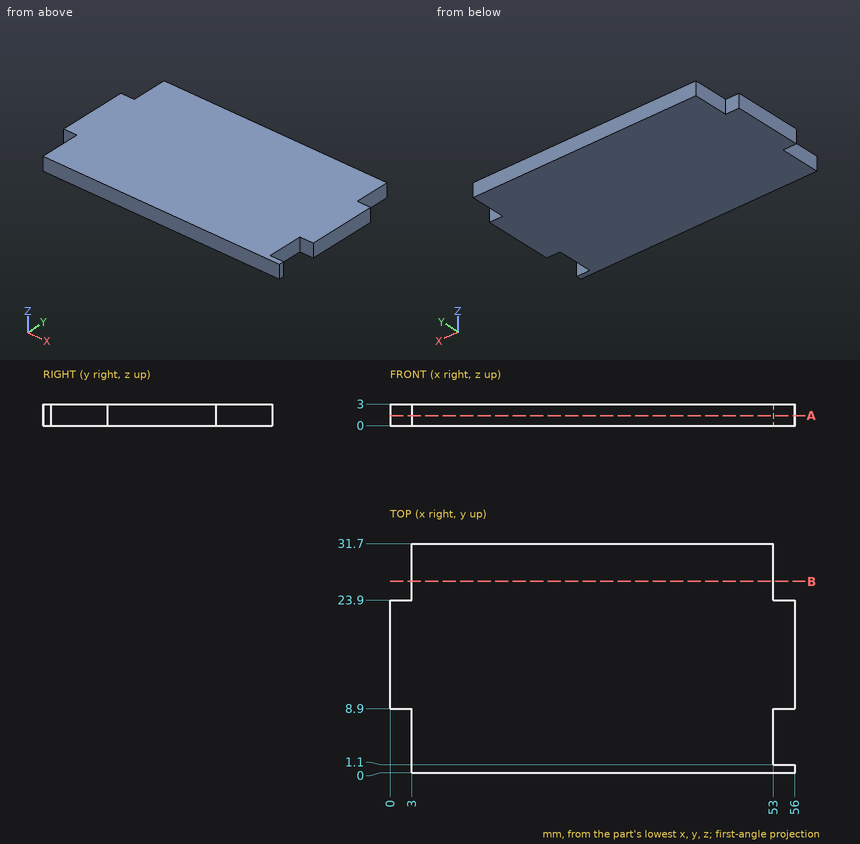
Geometry: see drawing. Coordinates: mm, zero at the bounding-box minimum. Give positions to 0.01 mm unless a question says otherwise; leave off trailing zeros. Write each loop counter-clockwise with the first axis right and the second up, starting at its lowest first coordinate (ties: lowest second). Pieces come first, ordered by that corner, then holes. Notation, with made-up numbers: (43.5, -0.75) -> (75.5, -0.75) arc R31 cw to (75.5, 24.25) -> close; hole circle Ø9 at (46, 4). An arc over 180 degrees is marked (long way). Use one line per item in the form item = value. Start each with the question number.
1) Pin query (flat end, axial travel): pin 1 (0.9 mm diameter, centred on y = 6.5, z = 1, fed in from -X); pin 2 (0.9 mm diameter, centred on x = 54, z = 1, fed in from +Y); pin 3 (1.5 mm diameter, centred on y = 24, z = 0.5, fed in from +X); pin 4 (1.5 mm diameter, centred on y = 6.5, z = 2, fed in from +X). Return the tip coordinate at first contact, or that it passes through.
2) Section query B-B on y = 26.5. Return the cut outline in (x, z), then the cut area to 3 significant figures.
3) Section query A-A on z = 1.4. Return the cut outline in (x, y).
4) Ray query, probe 1 along X at (y, z) = (7.5, 1.95). Return the intervals inside material, ascending. Write a range as from..to.
Outcome:
q1.pin_1 = 3
q1.pin_2 = 23.9
q1.pin_3 = 56
q1.pin_4 = 53
q2.outline = (3, 0) -> (53, 0) -> (53, 3) -> (3, 3) -> close
q2.area = 150 mm^2
q3.outline = (0, 8.9) -> (3, 8.9) -> (3, 0) -> (56, 0) -> (56, 1.1) -> (53, 1.1) -> (53, 8.9) -> (56, 8.9) -> (56, 23.9) -> (53, 23.9) -> (53, 31.7) -> (3, 31.7) -> (3, 23.9) -> (0, 23.9) -> close
q4.probe_1 = 3..53
